CAD build for the part. Positions are in the model's coordinates, mm. Give positions to 0.01 mm unless a question says otherwise; leave off trailing zeros. Loops run counter-clockwise (first coordinate to the right, second up) from the corner with the lowest first, then second, coordinate; pieces in that order, holes last. Notation, with made-up numbers: M 16,39.25 L 51,39.25 A19 ccw 51,63.25 Z; hole C -12.5,49.5 d2. An arc over 180 degrees is marked long. One line per question, with ' | ' between items.
```python
from build123d import *

# Parameters (mm, degrees)
ESBO_O1_R                = 32
ESBO_O1_R_2              = 5
ESBO_O1_R_3              = 3
RESSALTO_EXTRUS_O1_DEPTH = 6
RESSALTO_EXTRUS_O3_START = -6
ESBO_O2_R                = 5
ESBO_O2_R_2              = 3
RESSALTO_EXTRUS_O3_DEPTH = 6


with BuildPart() as part:
    # Esboço1 → Ressalto-extrusão1 (new body)
    with BuildSketch(Plane(origin=(0, 0, 0), x_dir=(1, 0, 0), z_dir=(0, 1, 0))):
        with Locations(Location((0, 0, 0), (0, 0, 270))):
            Circle(ESBO_O1_R)
        with Locations(Location((0, 0, 0), (0, 0, 270))):
            Circle(ESBO_O1_R_2, mode=Mode.SUBTRACT)
        with Locations(Location((0, 27, 0), (0, 0, 270))):
            Circle(ESBO_O1_R_3, mode=Mode.SUBTRACT)
        with Locations(Location((27, 0, 0), (0, 0, 270))):
            Circle(ESBO_O1_R_3, mode=Mode.SUBTRACT)
        with Locations(Location((0, -27, 0), (0, 0, 270))):
            Circle(ESBO_O1_R_3, mode=Mode.SUBTRACT)
        with Locations(Location((-27, 0, 0), (0, 0, 270))):
            Circle(ESBO_O1_R_3, mode=Mode.SUBTRACT)
        with Locations(Location((-19.091883092, 19.091883092, 0), (0, 0, 270))):
            Circle(ESBO_O1_R_3, mode=Mode.SUBTRACT)
        with Locations(Location((19.091883092, -19.091883092, 0), (0, 0, 270))):
            Circle(ESBO_O1_R_3, mode=Mode.SUBTRACT)
    extrude(amount=RESSALTO_EXTRUS_O1_DEPTH)

    # Esboço2 → Ressalto-extrusão3 (add)
    with BuildSketch(Plane(origin=(0, 6, 0), x_dir=(1, 0, 0), z_dir=(0, 1, 0)).offset(RESSALTO_EXTRUS_O3_START)):
        Circle(ESBO_O2_R)
        with Locations(Location((0, 0, 0), (0, 0, 270))):
            Circle(ESBO_O2_R_2, mode=Mode.SUBTRACT)
    extrude(amount=RESSALTO_EXTRUS_O3_DEPTH)


solid = part.part
```
Item 1: Saw through at C-C on x = -27. Give the cut face in (y, z), and give its area (3 significant figures).
Conclusion:
outline: M 0,-17.18 L 6,-17.18 L 6,-3 L 0,-3 Z; M 0,3 L 6,3 L 6,17.18 L 0,17.18 Z | area: 170 mm²
Item 2: Mould opens along Z. For faces 1 (the cylindrical face through (-31.24, 2.96, -6.94)), 2 (the flat face through (0, 0, 7)), 3 (the cylindrical face through (16.163, 2.958, 18.442)) say: pulls with the +Z half, pulls with the -Z half, needs draft (parallel to the pull), parting line crosses it, or undercut.
Conclusion:
face 1: parting line crosses it | face 2: needs draft | face 3: undercut
Item 3: Drop a flat-ended pin along its axis: P1, Ø1, axis at y = 2, z = 0, coming from the -X side. Give the stop position or say it passes through.
Conclusion:
P1: x = -32
Item 4: Saw through at B-B on x = 0. Give the cut face in (y, z), and give its area (3 significant figures).
Conclusion:
outline: M 0,-32 L 6,-32 L 6,-30 L 0,-30 Z; M 0,-24 L 6,-24 L 6,-3 L 0,-3 Z; M 0,3 L 6,3 L 6,24 L 0,24 Z; M 0,30 L 6,30 L 6,32 L 0,32 Z | area: 276 mm²
Item 5: Saw through at A-A on z = 0. Give the cut face in (x, y), and give its area (3 significant figures).
Conclusion:
outline: M -32,0 L -30,0 L -30,6 L -32,6 Z; M -24,0 L -3,0 L -3,6 L -24,6 Z; M 3,0 L 24,0 L 24,6 L 3,6 Z; M 30,0 L 32,0 L 32,6 L 30,6 Z | area: 276 mm²
Item 6: Saw through at D-D on z = 27. Give the cut face in (x, y), and give its area (3 significant figures).
Conclusion:
outline: M -17.18,0 L -3,0 L -3,6 L -17.18,6 Z; M 3,0 L 17.18,0 L 17.18,6 L 3,6 Z | area: 170 mm²
Item 7: Drill centre lines: line 1 along X through (y, z) = (3.25, 0); line 2 along X through (y, z) = (3.5, 16.5); line 3 along X through (y, z) = (3.2, -17). Where is each one in solid material? Low to high. Write a range as [from, to].
Conclusion:
line 1: [-32, -30], [-24, -3], [3, 24], [30, 32] | line 2: [-27.42, 17.58], [20.6, 27.42] | line 3: [-27.11, -21.24], [-16.94, 27.11]
